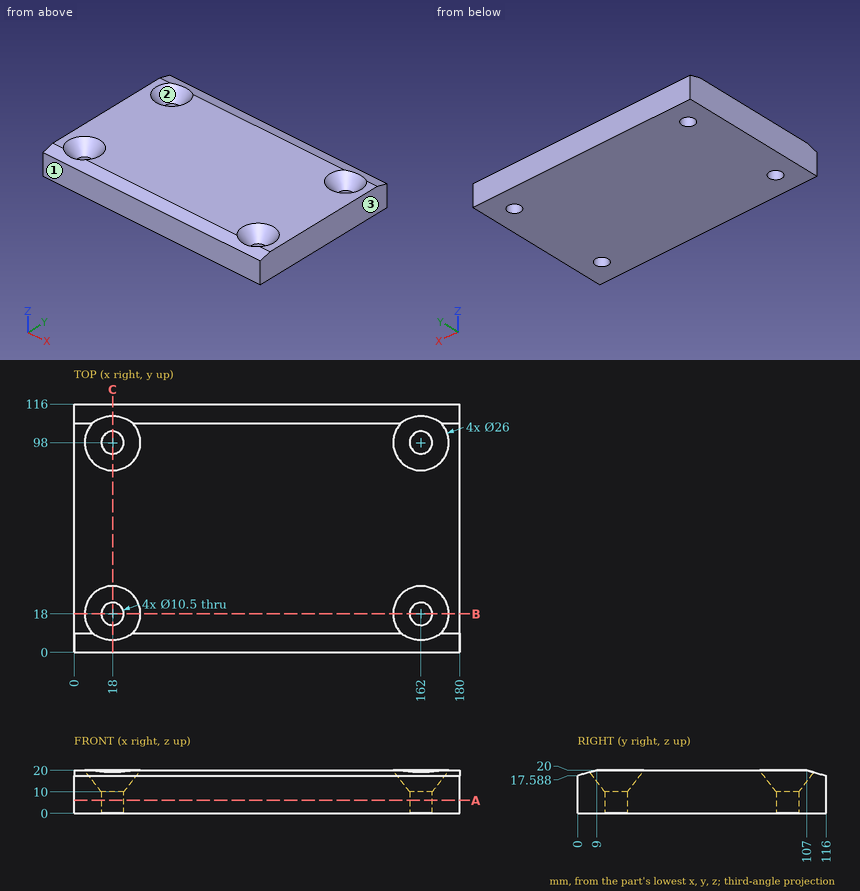
Check sheet for the drawn part. Datum: minimum x, y, z corner. Units: mm. Give positions to 0.01 mm unless a question says otherwise; leave off trailing zeros. Write each loop counter-clockwise with the first axis right and the second up, starting at its lowest first coordinate (ties: lowest second). Pieces come first, ordered by that corner, then holes. Notation, with made-up numbers: (38, 58) - (51, 58) arc R25 ccw to (51, 80) - close; hole circle Ø6 at (-6, 19). An arc over 180 degrees is marked (long way). Put each result on its own line as item: value.
1. Thickness scan on line 1 (Y direction, x = 162, z = 5.5); line 2 (X direction, y = 92.5, z = 15.75) (1 decimal); line 3 (Y direction, x = 22, z = 4.5). Record the ranges inside material, lowest first.
Ans:
line 1: y = 0 to 12.75, 23.25 to 92.75, 103.25 to 116
line 2: x = 0 to 10, 26 to 154, 170 to 180
line 3: y = 0 to 14.6, 21.4 to 94.6, 101.4 to 116
2. Go/stop test with flat-tipped pins: pin 1 (4 mm diameter, centred on x = 88, z = 2.5, fed in from -Y); pin 2 (6.5 mm diameter, centred on x = 18, y = 98, fed in from -Z) (3 decimals); pin 3 (13.5 mm diameter, centred on x = 18, y = 18, fed in from +Z) (1 decimal). Record where each tip stops, or that it passes through.
Ans:
pin 1: stops at y = 0
pin 2: passes through
pin 3: stops at z = 11.9
3. Draft check along Y on the marked faces 1, 2 and 3. Enter one of: +Y half, -Y half, draft (parallel to the pull), parting line (faces both ways), or undercut.
Ans:
face 1: -Y half
face 2: undercut
face 3: draft
4. Sectioned sample at A-A, the plane z = 6. Enter the section's corners in (x, y), plus the area to 3 significant figures.
Ans:
outline: (0, 0) - (180, 0) - (180, 116) - (0, 116) - close; hole circle Ø10.5 at (18, 18); hole circle Ø10.5 at (18, 98); hole circle Ø10.5 at (162, 18); hole circle Ø10.5 at (162, 98)
area: 20,500 mm²
5. Sectioned sample at C-C, the plane x = 18. Enter the section's corners in (y, z), plus the area to 3 significant figures.
Ans:
outline: (0, 0) - (12.75, 0) - (12.75, 10) - (5.69, 19.11) - (0, 17.59) - close; (23.25, 0) - (92.75, 0) - (92.75, 10) - (85, 20) - (31, 20) - (23.25, 10) - close; (103.25, 0) - (116, 0) - (116, 17.59) - (110.31, 19.11) - (103.25, 10) - close
area: 1,730 mm²
6. Sectioned sample at B-B, the plane y = 18. Enter the section's corners in (x, z), plus the area to 4 significant figures.
Ans:
outline: (0, 0) - (12.75, 0) - (12.75, 10) - (5, 20) - (0, 20) - close; (23.25, 0) - (156.75, 0) - (156.75, 10) - (149, 20) - (31, 20) - (23.25, 10) - close; (167.25, 0) - (180, 0) - (180, 20) - (175, 20) - (167.25, 10) - close
area: 3,025 mm²
